Autodesk Inventor part; units mm, degrees
ref_plane "YZ Plane" through (0, 0, 0) normal (1, 0, 0) x (0, 1, 0)
ref_plane "XZ Plane" through (0, 0, 0) normal (0, 1, 0) x (-1, 0, 0)
ref_plane "XY Plane" through (0, 0, 0) normal (0, 0, 1) x (1, 0, 0)
sketch "スケッチ1" plane through (0, 0, 0) normal (0, 0, 1) x (1, 0, 0)
  circle A0 centre (0, 0) radius 4
  dimension "d0" = 8
extrude "押し出し1" add sketch "スケッチ1" against normal blind 155
sketch "スケッチ2" plane through (0, 0, -155) normal (0, 0, -1) x (-1, 0, 0)
  circle A0 centre (0, 0) radius 3
  dimension "d3" = 6
extrude "押し出し2" add sketch "スケッチ2" along normal blind 26
sketch "スケッチ3" plane through (0, 0, 0) normal (0, 0, 1) x (1, 0, 0)
  circle A0 centre (0, 0) radius 9.5613
extrude "押し出し3" cut sketch "スケッチ3" against normal blind 40
properties part number "円柱8mm" material "ステンレス鋼"
Model file for the job. Use its own axes, mm. A direction names the side the tool comes from. Coordinates: 2 decimals unless noted, no trailing zeros. Order: outer loops, then holes, each group sorted by start corner. A loop starts at its lowest first (then second) coordinate and runs counter-clockwise, first axis right, second up. Notation, with made-up numbers: (-36, 57.25) -> (-2, 57.25) arc R18 cw to (-2, 85.25) -> close; hole circle Ø6 at (49.5, 62). An arc over 180 degrees is marked (long way). Answer as a JSON object with one key per item and string values. Group by question number.
1) Cut at D-D, the plane z = -169.5. Write the cut outline in (x, y), then the cut area to 3 significant figures.
2) Flat gauge pins, fed straight in: pin 1 (1.5 mm diameter, centred on x = -3, z = -62.5, fed in from +Y); pin 2 (1.5 mm diameter, centred on y = -2.5, z = -157, fed in from -X); pin 3 (1.5 mm diameter, centred on x = 2, z = -163.5, fed in from -Y). Where does each tip first touch, or does it go through?
3) Drill centre lines: L1, parallel to Z at x = -1.25, y = -3; L2, parallel to Y at x = -0.25, z = -146.5; L3, parallel to X at y = 0.5, z = -137. Where is each one in solid material? Low to high.
4) Cut at A-A, the plane x = 0. Write the cut outline in (y, z), then the cut area to 3 significant figures.
5) Which spindle directions (+Z, -Z, +X, -X, +Y, -Y) get a long thin tool onto all of the face, cutting with end or side? Do faces 1 (the face through (3, 0, -168)), 2 (the face through (-0.867, -3.905, -96.695)). Say none if no direction does.
6) Cut at C-C, the plane z = -147. Write the cut outline in (x, y).
Check values:
{
 "1": {"outline": "circle Ø6 at (0, 0)", "area": "28.3 mm²"},
 "2": {"pin 1": "stops at y = 3.31", "pin 2": "stops at x = -2.44", "pin 3": "stops at y = -2.73"},
 "3": {"L1": "z = -155 to -40", "L2": "y = -3.99 to 3.99", "L3": "x = -3.97 to 3.97"},
 "4": {"outline": "(-4, -155) -> (-3, -155) -> (-3, -181) -> (3, -181) -> (3, -155) -> (4, -155) -> (4, -40) -> (-4, -40) -> close", "area": "1,080 mm²"},
 "5": {"face 1": "-Z", "face 2": "+Z, -Z"},
 "6": {"outline": "circle Ø8 at (0, 0)"}
}
